```python
from build123d import *

# Parameters (mm, degrees)
REVOLVE2_ANGLE        = 180
CUT_EXTRUDE1_DEPTH    = 50
F_2_0MM_DOWEL_HOLE1_D = 2.3
SKETCH13_R            = 1.65
CUT_EXTRUDE2_DEPTH    = 100


with BuildPart() as part:
    # Sketch3 → Revolve2 (revolve)
    with BuildSketch(Plane.XY):
        Polygon((48.25, 0), (47.584421203, -12.7), (55, -12.7), (55, 0), align=None)
    revolve(axis=Axis((0, 50.355486862, 0), (0, -1, 0)), revolution_arc=REVOLVE2_ANGLE)

    # Sketch9 → Cut-Extrude1 (cut)
    with BuildSketch(Plane.XY.offset(55)):
        Polygon((53.725, -4.562435565), (53.725, -2.137564435), (51.625, -0.925128869), (49.525, -2.137564435), (49.525, -4.562435565), (51.625, -5.774871131), align=None)
        Polygon((53.725, -10.562435565), (53.725, -8.137564435), (51.625, -6.925128869), (49.525, -8.137564435), (49.525, -10.562435565), (51.625, -11.774871131), align=None)
    cut_extrude1 = extrude(amount=-CUT_EXTRUDE1_DEPTH, mode=Mode.SUBTRACT)

    # Ø2.0mm Dowel Hole1 (through all)
    with Locations(Plane.XY.offset(5)):
        with Locations((51.625, -9.35), (51.625, -3.35)):
            f_2_0mm_dowel_hole1 = Hole(F_2_0MM_DOWEL_HOLE1_D / 2)

    # Mirror2: Cut-Extrude1, Ø2.0mm Dowel Hole1 across plane
    add(cut_extrude1.mirror(Plane(origin=(0, 0, 0), x_dir=(0, 0, 1), z_dir=(1, 0, 0))), mode=Mode.SUBTRACT)
    add(f_2_0mm_dowel_hole1.mirror(Plane(origin=(0, 0, 0), x_dir=(0, 0, 1), z_dir=(1, 0, 0))), mode=Mode.SUBTRACT)

    # Sketch13 → Cut-Extrude2 (cut, symmetric)
    with BuildSketch(Plane(origin=(0, 0, 0), x_dir=(0.707106781, 0, 0.707106781), z_dir=(-0.707106781, 0, 0.707106781))):
        with Locations((0, -6.35)):
            Circle(SKETCH13_R)
    extrude(amount=CUT_EXTRUDE2_DEPTH, both=True, mode=Mode.SUBTRACT)


solid = part.part
```
Part model, mm, in its own coordinate system. A direction names the side the tool comes from. Round coordinates to 2 decimals unless told otherwise and drop trailing zeros. Loops run counter-clockwise (first coordinate to the right, second up) from the corner with the lowest first, then second, coordinate; pieces in that order, holes last.
Item 1: Drill centre lines: line 1 (X direction, y = -5.75, z = 28); line 2 (X direction, y = -2.25, z = 29); line 3 (Z direction, x = -24.5, y = -6.5). Where is each one in solid material? Low to high.
Item 2: Cut at A-A, the plane y = -3.35. Give the cut face in (x, z) (3 decimals), then the cut area to 3 significant figures.
Item 3: Cut at C-C, the plane y = -9.35. Give the cut face in (x, z) (3 decimals), then the cut area to 3 significant figures.
Item 4: Drop flat-ended pins along their axis: P1, Ø1, axis at y = -2, z = 35.5, coming from the -X side; P2, Ø2.5, axis at y = -3.5, z = 10, coming from the -X side; P3, Ø1.2, axis at y = -9, z = 7, coming from the +X side; P4, Ø1.3, axis at x = 51.5, y = -9.5, coming from the +Z side. Give the stop position or say it passes through.
Item 5: Cut at B-B, the plane x = 0. Give the cut face in (y, z).
Item 6: 3-axis set-ups, long thin cutter, end or side, ignore diameter. For faces 1 (the face through (-50.56, -5.16, 12.49)), 2 (the face through (-51, -6, 0)): which of +Z, -Z, +X, -X, +Y, -Y reach the whole face in a straight line?
A:
1. line 1: x = -47.34 to -38.92, 38.92 to 47.34
1. line 2: x = -46.73 to -38.41, 38.41 to 46.73
1. line 3: z = 41.17 to 49.24
2. outline: (-55, 0) - (-52.775, 0) - (-52.775, 5) - (-53.725, 5) - (-53.725, 11.774) arc R55 ccw to start; (-50.475, 0) - (-48.074, 0) arc R48.074 cw to (48.074, 0) - (50.475, 0) - (50.475, 5) - (49.525, 5) - (49.525, 23.922) arc R55 ccw to (-49.525, 23.922) - (-49.525, 5) - (-50.475, 5) - close; (52.775, 0) - (55, 0) arc R55 ccw to (53.725, 11.774) - (53.725, 5) - (52.775, 5) - close
2. area: 984 mm2
3. outline: (-55, 0) - (-52.775, 0) - (-52.775, 5) - (-53.725, 5) - (-53.725, 11.774) arc R55 ccw to start; (-50.475, 0) - (-47.76, 0) arc R47.76 cw to (47.76, 0) - (50.475, 0) - (50.475, 5) - (49.525, 5) - (49.525, 23.922) arc R55 ccw to (-49.525, 23.922) - (-49.525, 5) - (-50.475, 5) - close; (52.775, 0) - (55, 0) arc R55 ccw to (53.725, 11.774) - (53.725, 5) - (52.775, 5) - close
3. area: 1,030 mm2
4. P1: stops at x = -42.43
4. P2: stops at x = -54.3
4. P3: stops at x = 54.63
4. P4: passes through
5. outline: (-12.7, 47.58) - (0, 48.25) - (0, 55) - (-12.7, 55) - close
6. face 1: +Z
6. face 2: -Z, +X, -X, +Y, -Y
